The model under review builds one solid part; all positions refer to its coordinate system, in mm. A direction names the side the tool comes from. Round coordinates to 2 decimals unless told otherwise and drop trailing zeros. Order: outer loops, then holes, each group sorted by start corner. A loop starts at its lowest first (then second) coordinate and runs counter-clockwise, first axis right, second up.
1) Clearance check with flat-ended pins moving along their axes: P1, Ø4, axis at x = -59.6, z = -7.6, coming from the -Y side; P2, Ø2, axis at x = 62, z = 0, coming from the -Y side. State where each tip first meets the part, or that it passes through.
2) To check wall thickness, follow L1, parallel to Z at x = -59.6, y = 1.5; L2, parallel to X at y = 1.4, z = -7.6; L3, parallel to X at y = 0.35, z = 6.75. State the ranges of each line that lie inside material, in increasing order.
3) Consider section B-B (z = 0). Give the boundary of the cut face in (x, y), then the cut area to 3 significant figures.
4) Consider section D-D (x = -4.5). Give the boundary of the cut face in (y, z), then the cut area to 3 significant figures.
5) Consider section C-C (y = 0.3). Give the number of separate pieces and of enclosed holes in the cut face, then the cut area to 3 significant figures.
6) Consider section A-A (x = -53). Give the boundary of the cut face in (y, z), then the cut area to 3 significant figures.
7) Machinability: for faces 1 (the face through (-1, 1, 13)), 2 (the face through (17, 1, -1.544)), which of the approach directions +Z, -Z, +X, -X, +Y, -Y give a long, thin tool a straight path to every point of the face, cutting with its end or side? Answer none if there is none.
8) Mouldability with a two-part tool opening along Z and no side actions: class faces 3 (the face through (-51.938, 0.986, 0.44)), 4 (the face through (64, 1, -11)), 5 (the face through (-64, 1, 11)), 6 (the face through (-65, 1, 0)) as pulls with the +Z half, pulls with the -Z half, needs draft (parallel to the pull), parting line crosses it, or undercut.
from build123d import *

# Parameters (mm, degrees)
ESBO_O1_R                = 1.6
ESBO_O1_R_2              = 1.15
RESSALTO_EXTRUS_O1_DEPTH = 2


with BuildPart() as part:
    # Esboço1 → Ressalto-extrusão1 (new body)
    with BuildSketch(Plane(origin=(0, 0, 0), x_dir=(1, 0, 0), z_dir=(0, 1, 0))):
        with BuildLine():
            Line((-60, -13), (60, -13))
            ThreePointArc((60, -13), (63.535533906, -11.535533906), (65, -8))
            Line((65, -8), (65, 8))
            ThreePointArc((65, 8), (63.535533906, 11.535533906), (60, 13))
            Line((60, 13), (-60, 13))
            ThreePointArc((-60, 13), (-63.535533906, 11.535533906), (-65, 8))
            Line((-65, 8), (-65, -8))
            ThreePointArc((-65, -8), (-63.535533906, -11.535533906), (-60, -13))
        make_face()
        with Locations((59.6, 7.6)):
            Circle(ESBO_O1_R, mode=Mode.SUBTRACT)
        with Locations((59.6, -7.6)):
            Circle(ESBO_O1_R, mode=Mode.SUBTRACT)
        with Locations((62, 0)):
            Circle(ESBO_O1_R_2, mode=Mode.SUBTRACT)
        with Locations((53, 0)):
            Circle(ESBO_O1_R_2, mode=Mode.SUBTRACT)
        with Locations((-59.6, 7.6)):
            Circle(ESBO_O1_R, mode=Mode.SUBTRACT)
        with Locations((-59.6, -7.6)):
            Circle(ESBO_O1_R, mode=Mode.SUBTRACT)
        with Locations((-53, 0)):
            Circle(ESBO_O1_R_2, mode=Mode.SUBTRACT)
        with Locations((-62, 0)):
            Circle(ESBO_O1_R_2, mode=Mode.SUBTRACT)
        with Locations((-44, 0)):
            Circle(ESBO_O1_R_2, mode=Mode.SUBTRACT)
        with BuildLine():
            Line((3.307143995, -1.544441193), (30.307143995, -1.544441193))
            Line((30.307143995, -1.544441193), (30.307143995, 1.544441193))
            Line((30.307143995, 1.544441193), (3.307143995, 1.544441193))
            ThreePointArc((3.307143995, 1.544441193), (0, 3.65), (-3.307143995, 1.544441193))
            Line((-3.307143995, 1.544441193), (-21.692856005, 1.544441193))
            Line((-21.692856005, 1.544441193), (-21.692856005, -1.544441193))
            Line((-21.692856005, -1.544441193), (-3.307143995, -1.544441193))
            ThreePointArc((-3.307143995, -1.544441193), (0, -3.65), (3.307143995, -1.544441193))
        make_face(mode=Mode.SUBTRACT)
    extrude(amount=RESSALTO_EXTRUS_O1_DEPTH)


solid = part.part
Answer below:
1. P1: stops at y = 0
1. P2: passes through
2. L1: z = -13 to -9.2, -6 to 6, 9.2 to 13
2. L2: x = -65 to -61.2, -58 to 58, 61.2 to 65
2. L3: x = -65 to -60.96, -58.24 to 58.24, 60.96 to 65
3. outline: (-65, 0) - (-63.15, 0) - (-63.15, 2) - (-65, 2) - close; (-60.85, 0) - (-54.15, 0) - (-54.15, 2) - (-60.85, 2) - close; (-51.85, 0) - (-45.15, 0) - (-45.15, 2) - (-51.85, 2) - close; (-42.85, 0) - (-21.69, 0) - (-21.69, 2) - (-42.85, 2) - close; (30.31, 0) - (51.85, 0) - (51.85, 2) - (30.31, 2) - close; (54.15, 0) - (60.85, 0) - (60.85, 2) - (54.15, 2) - close; (63.15, 0) - (65, 0) - (65, 2) - (63.15, 2) - close
3. area: 133 mm2
4. outline: (0, -13) - (2, -13) - (2, -1.54) - (0, -1.54) - close; (0, 1.54) - (2, 1.54) - (2, 13) - (0, 13) - close
4. area: 45.8 mm2
5. separate pieces: 1
5. enclosed holes: 10
5. area: 3,120 mm2
6. outline: (0, -13) - (2, -13) - (2, -1.15) - (0, -1.15) - close; (0, 1.15) - (2, 1.15) - (2, 13) - (0, 13) - close
6. area: 47.4 mm2
7. face 1: +Z, +X, -X, +Y, -Y
7. face 2: +Y, -Y
8. face 3: undercut
8. face 4: pulls with the -Z half
8. face 5: pulls with the +Z half
8. face 6: needs draft
